For this review, take the finished solid that the model builds, in its own axes (mm). Give positions to 0.01 mm unless a question says otherwise; leave off trailing zeros. Order: outer loops, then holes, each group sorted by start corner. A loop starts at its lowest first (then second) coordinate and runs counter-clockwise, first axis right, second up. Notation, with made-up numbers: (6, 77.5) - (39, 77.5) arc R17 ccw to (39, 89.5) - close; hole circle Ø1 at (14.5, -12.5). An arc over 180 degrees is marked (long way). Put each result on its own line as item: value. Start each with the question number.
```python
from build123d import *

# Parameters (mm, degrees)
EXTRUDE_1_DEPTH          = 50
EXTRUDE_1_DEPTH_BACK     = 50
SKETCH_1_R               = 50
CUT_EXTRUDE_2_DEPTH      = 50
CUT_EXTRUDE_2_DEPTH_BACK = 50
SKETCH_2_R               = 40
EXTRUDE_2_REACH          = 225.861
EXTRUDE_2_END_RADIUS     = 50
SKETCH_3_R               = 40


with BuildPart() as part:
    # Sketch 1 → Extrude 1 (new, two sides: drawn at the far end of the back side and taken through both)
    with BuildSketch(Plane(origin=(0, 0, 0), x_dir=(0, 0, -1), z_dir=(1, 0, 0)).offset(-EXTRUDE_1_DEPTH_BACK)):
        Circle(SKETCH_1_R)
    extrude(amount=EXTRUDE_1_DEPTH + EXTRUDE_1_DEPTH_BACK)

    # Sketch 2 → Cut-Extrude 2 (cut, two sides: drawn at the far end of the back side and taken through both)
    with BuildSketch(Plane(origin=(0, 0, 0), x_dir=(0, 0, -1), z_dir=(1, 0, 0)).offset(-CUT_EXTRUDE_2_DEPTH_BACK)):
        Circle(SKETCH_2_R)
    extrude(amount=CUT_EXTRUDE_2_DEPTH + CUT_EXTRUDE_2_DEPTH_BACK, mode=Mode.SUBTRACT)

    # Extrude 2: up to this cylinder (the profile starts outside it)
    extrude_2_end = Plane(origin=(0, 0, 0), z_dir=(-1, 0, 0)) * Cylinder(EXTRUDE_2_END_RADIUS, 552.722, mode=Mode.PRIVATE)
    # Sketch 3 → Extrude 2 (add, up to the surface)
    with BuildSketch(Plane(origin=(0, -162.4, 0), x_dir=(-1, 0, 0), z_dir=(0, -1, 0)), mode=Mode.PRIVATE) as extrude_2_sk1:
        with Locations(Location((0, 0, 0), (0, 0, 180))):
            Circle(SKETCH_3_R)
    extrude_2_tool1 = extrude(extrude_2_sk1.sketch, amount=-EXTRUDE_2_REACH, mode=Mode.PRIVATE) - extrude_2_end
    add(extrude_2_tool1.solids().sort_by_distance((0, -162.4, 0))[0])


solid = part.part
```
1. Add section D-D, the plane z = 20. Give the boundary of the cut face in (x, y).
2. Add section A-A, the plane z = 0. Give the boundary of the cut face in (x, y), then the cut area to 3 significant figures.
3. Clearance check with flat-ended pins moving along their axes: pin 1 (8 mm diameter, centred on x = 23, y = -90.5, fed in from +Z); pin 2 (10 mm diameter, centred on y = -90.5, z = 16.5, fed in from +X); pin 3 (6 mm diameter, centred on x = -14, y = -35, fed in from +Z). State where each tip first meets the part, or that it passes through.
4. Wall thickness on line 1 (Y direction, x = -8, z = 0); line 2 (Y direction, x = 32, z = -8.5); line 3 (Z direction, x = -9.5, y = -34): over which ranges is each line inside the solid? List them lowest first. Write a range as from..to.
5. The part is to be moulded in two halves that separate along Z. For faces 1 (the face through (38.153, -97.127, 12.015)), 2 (the face through (-50, 34, 22)), 3 (the face through (-0.7, -39.05, 8.67)), say which applies: released by +Z, released by -Z, zero draft, split by the parting line, or undercut.
6. Add section C-C, the plane x = 0. Give the boundary of the cut face in (y, z), then the cut area to 3 significant figures.
7. Add section B-B, the plane y = 0. Give the boundary of the cut face in (x, z), then the cut area to 3 significant figures.
Found:
1. outline: (-50, -45.83) - (-34.64, -45.83) - (-34.64, -162.4) - (34.64, -162.4) - (34.64, -45.83) - (50, -45.83) - (50, -34.64) - (-50, -34.64) - close; (-50, 34.64) - (50, 34.64) - (50, 45.83) - (-50, 45.83) - close
2. outline: (-50, -50) - (-40, -50) - (-40, -162.4) - (40, -162.4) - (40, -50) - (50, -50) - (50, -40) - (-50, -40) - close; (-50, 40) - (50, 40) - (50, 50) - (-50, 50) - close
2. area: 11,000 mm^2
3. pin 1: stops at z = 35.2
3. pin 2: stops at x = 38.31
3. pin 3: stops at z = 38.46
4. line 1: y = -162.4..-40, 40..50
4. line 2: y = -162.4..-39.09, 39.09..49.27
4. line 3: z = -38.86..-21.07, 21.07..38.86
5. face 1: split by the parting line
5. face 2: zero draft
5. face 3: undercut
6. outline: (-162.4, -40) - (-30, -40) arc R50 ccw (long way) to (-30, 40) - (-162.4, 40) - close; hole circle Ø80 at (0, 0)
6. area: 12,300 mm^2
7. outline: (-50, -50) - (50, -50) - (50, -40) - (-50, -40) - close; (-50, 40) - (50, 40) - (50, 50) - (-50, 50) - close
7. area: 2,000 mm^2
